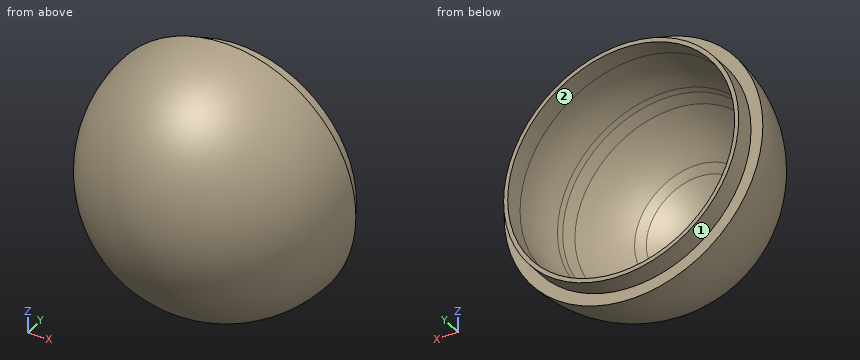
from build123d import *


with BuildPart() as part:
    # Sketch1 → Revolve2 (revolve)
    with BuildSketch(Plane.XY, mode=Mode.PRIVATE) as revolve2_sk:
        with BuildLine():
            Line((0, -25), (0, -28.503418665))
            ThreePointArc((0, -28.503418665), (-20.154960625, -20.154960625), (-28.503418665, 0))
            Line((-28.503418665, 0), (-25.9, 0))
            Line((-25.9, 0), (-25.9, 2))
            Line((-25.9, 2), (-25.9, 2.5))
            Line((-25.9, 2.5), (-25.9, 4.3))
            Line((-25.9, 4.3), (-25, 4.3))
            Line((-25, 4.3), (-25, 0))
            ThreePointArc((-25, 0), (-24.490431494, -5.021828876), (-22.982498779, -9.838940484))
            ThreePointArc((-22.982498779, -9.838940484), (-22.747404845, -10.37090029), (-22.5, -10.897247359))
            ThreePointArc((-22.5, -10.897247359), (-21.902104859, -12.053953822), (-21.244795494, -13.177961315))
            ThreePointArc((-21.244795494, -13.177961315), (-17.691022269, -17.664306696), (-13.210052688, -21.2248559))
            ThreePointArc((-13.210052688, -21.2248559), (-12.26215849, -21.786222003), (-11.29045343, -22.305283261))
            ThreePointArc((-11.29045343, -22.305283261), (-5.803788352, -24.316990783), (0, -25))
        make_face()
    revolve(revolve2_sk.sketch.rotate(Axis((0, -29.246756477, 0), (0, 1, 0)), 180), axis=Axis((0, -29.246756477, 0), (0, 1, 0)))


solid = part.part
CAD build for the part. Positions are in the model's coordinates, mm. Face numbers are marked on the shaded views. Round coordinates to 2 decimals unless told otherwise and drop trailing zeros. Order: outer loops, then holes, each group sorted by start corner. A loop starts at its lowest first (then second) coordinate and runs counter-clockwise, first axis right, second up. Notation, with made-up numbers: (23.5, -7.75) - (80.5, -7.75) arc R29 cw to (80.5, 25.25) - close; hole circle Ø5 at (16, 77). An arc over 180 degrees is marked (long way). Return JSON: item names as keys, results as strings.
(1) Pull direction Z, two halves, no side cores. Call the marked faces 1 and 2: +Z half, -Z half, draft (parallel to the pull), parting line (faces both ways), or undercut.
Answer key:
{"face 1": "parting line", "face 2": "undercut"}
(2) Pin check, flat tips, straight feed: pin 1 Ø4 at (x, y) = (6.5, -22.5) entering from -Z; pin 2 Ø5 at (y, z) = (-15.5, 8) entering from -X; pin 3 Ø1.5 at (x, z) = (-11.5, 16.5) entering from -Y. Stop position of each tip, or through.
Answer key:
{"pin 1": "stops at z = -18.8", "pin 2": "stops at x = -24.27", "pin 3": "stops at y = -20.92"}
(3) Wall check: probe 1 along Z at (x, y) = (0, 3); probe 2 along Z at (x, y) = (8.5, -21.5); probe 3 along X at (y, z) = (-11, 8). Give the ranges that are in metal, low to high. Write a range as from..to.
Answer key:
{"probe 1": "z = -25.9..-25, 25..25.9", "probe 2": "z = -16.67..-9.51, 9.51..16.67", "probe 3": "x = -25.05..-20.98, 20.98..25.05"}
(4) Cut at A-A (y = -19.5). Give the cut face in (x, z), then the cut area to 3 significant figures.
Answer key:
{"outline": "circle Ø41.58 at (0, 0); hole circle Ø31.29 at (0, 0)", "area": "589 mm^2"}
